Part model, mm, in its own coordinate system. A direction names the side the tool comes from. Give positions to 0.01 mm unless a question says otherwise; leave off trailing zeros. Loops run counter-clockwise (first coordinate to the right, second up) from the corner with the lowest first, then second, coordinate; pieces in that order, holes last. Notation, with made-up numbers: M -24,27 L 28,27 A8 cw 28,31 Z; hole C 74,-10 d9. An arc over 180 degrees is marked long. Put each result on its own line as item: value. Start each with the question number.
```python
from build123d import *

# Parameters (mm, degrees)
SKETCH2_R           = 2.1
BOSS_EXTRUDE2_DEPTH = 4
SKETCH3_W           = 2
SKETCH3_H           = 9.2
BOSS_EXTRUDE3_DEPTH = 4


with BuildPart() as part:
    # Sketch2 → Boss-Extrude2 (new body)
    with BuildSketch(Plane.XY):
        with BuildLine():
            Line((0, 4.6), (37, 4.6))
            Line((37, 4.6), (37, -4.6))
            Line((37, -4.6), (0, -4.6))
            ThreePointArc((0, -4.6), (-4.6, 0), (0, 4.6))
        make_face()
        Circle(SKETCH2_R, mode=Mode.SUBTRACT)
    extrude(amount=BOSS_EXTRUDE2_DEPTH)

    # Sketch3 → Boss-Extrude3 (add)
    with BuildSketch(Plane.XY.offset(4)):
        with Locations((36, 0)):
            Rectangle(SKETCH3_W, SKETCH3_H)
        with BuildLine():
            Line((1.9, 4.6), (1.9, 0.894427191))
            ThreePointArc((1.9, 0.894427191), (-2.1, 0), (1.9, -0.894427191))
            Line((1.9, -0.894427191), (1.9, -4.6))
            Line((1.9, -4.6), (0, -4.6))
            ThreePointArc((0, -4.6), (-4.6, 0), (0, 4.6))
            Line((0, 4.6), (1.9, 4.6))
        make_face()
    extrude(amount=BOSS_EXTRUDE3_DEPTH)


solid = part.part
```
1) Which spindle directions (+Z, -Z, +X, -X, +Y, -Y) get a long thin tool onto all of the face, cutting with end or side? Do faces 4 (the flat face through (1.9, -3, 6)), 5 (the flat face through (16, 0, 0)). Say none if no direction does.
2) Wall check: L1, parallel to Y at x = 0, z = 4; L2, parallel to X at y = 0, z = 3.75; L3, parallel to X at y = 0, z = 6. Give the ranges that are in metal, low to high.
3) Mould opens along X. For faces 1 (the flat face through (1.9, 3, 6)), 2 (the flat face through (37, 0, 4)), 3 (the flat face through (18, -4.6, 2)) say: +X half, -X half, draft (parallel to the pull), parting line (faces both ways), or undercut.
4) Band-saw the part on D-D on x = 30. Give the cut face in (y, z), then the cut area to 3 significant figures.
5) Band-saw the part on B-B on y = 0. Give the cut face in (x, z), then the cut area to 3 significant figures.
6) Band-saw the part on A-A on z = 7. Give the cut face in (x, y), then the cut area to 3 significant figures.
7) Band-saw the part on C-C on z = 1.5. Give the cut face in (x, y).
8) Pin check, flat tip, straight feed: pin 1 Ø1.5 at (y, z) = (1, 1) entering from -X. Stop position of the tip, or through.
Evaluation:
1. face 4: +Z, +Y, -Y
1. face 5: -Z, +X, -X, +Y, -Y
2. L1: -4.6 to -2.1, 2.1 to 4.6
2. L2: -4.6 to -2.1, 2.1 to 37
2. L3: -4.6 to -2.1, 35 to 37
3. face 1: undercut
3. face 2: +X half
3. face 3: draft
4. outline: M -4.6,0 L 4.6,0 L 4.6,4 L -4.6,4 Z
4. area: 36.8 mm2
5. outline: M -4.6,0 L -2.1,0 L -2.1,8 L -4.6,8 Z; M 2.1,0 L 37,0 L 37,8 L 35,8 L 35,4 L 2.1,4 Z
5. area: 168 mm2
6. outline: M 0,-4.6 L 1.9,-4.6 L 1.9,-0.89 A2.1 cw long 1.9,0.89 L 1.9,4.6 L 0,4.6 A4.6 ccw Z; M 35,-4.6 L 37,-4.6 L 37,4.6 L 35,4.6 Z
6. area: 55.5 mm2
7. outline: M 0,-4.6 L 37,-4.6 L 37,4.6 L 0,4.6 A4.6 ccw Z; hole C 0,0 d4.2
8. pin 1: x = -4.59
